Model file for the job. Use its own axes, mm. A direction names the side the tool comes from. Coordinates: 2 decimals unless noted, no trailing zeros. Order: outer loops, then holes, each group sorted by start corner. A loop starts at its lowest first (then second) coordinate and runs counter-clockwise, first axis right, second up. Notation, with made-up numbers: (59.5, 53) -> (66.5, 53) arc R25 ccw to (66.5, 71) -> close; hole circle Ø2 at (19, 50). An arc over 180 degrees is marked (long way). Use CSV: the item, a comma, the result in double quotes. Start each with the question number.
(1) Tool access for faces 1 (the cylindrical face through (-264, -40, 9)), 2 (the cylindrical face through (363.235, 38.668, 5.077)), 3 (the cylindrical face through (3.08, 2.64, 59.94)): list every direction of +Z, -Z, +X, -X, +Y, -Y with a clear straight run to the whole face (end or side of a thin tool).
(2) Probe L1, parallel to Y at x = 415, z = 0; L2, parallel to X at y = 4, z = -41; L3, parallel to Y at x = 417.25, z = 0. List the from-to ranges inside material, lowest first.
(3) Cut at B-B on x = 81.5. Write the cut outline in (y, z).
(4) Pin check, flat tips, straight feed: pin 1 Ø8 at (x, y) = (3, 16) entering from -Z; pin 2 Ø3 at (x, y) = (-96.5, -11.5) entering from -Z; pin 3 Ø5 at (x, z) = (-42, 21.5) entering from +Y. Stop position of each tip, or through.
(5) Cut at A-A on x = 280. Write the cut outline in (y, z).
```python
from build123d import *

# Parameters (mm, degrees)
SKETCH1_R           = 60
BOSS_EXTRUDE1_DEPTH = 220
SKETCH2_R           = 41
BOSS_EXTRUDE2_DEPTH = 310
SKETCH3_R           = 39
BOSS_EXTRUDE3_DEPTH = 420
SKETCH4_R           = 3.75
CUT_EXTRUDE1_DEPTH  = 6.25
SKETCH5_R           = 3.6
CUT_EXTRUDE2_DEPTH  = 6.25
CHAMFER1_SIZE       = 5


with BuildPart() as part:
    # Sketch1 → Boss-Extrude1 (new body, symmetric)
    with BuildSketch(Plane(origin=(0, 0, 0), x_dir=(0, 0, -1), z_dir=(1, 0, 0))):
        Circle(SKETCH1_R)
    extrude(amount=BOSS_EXTRUDE1_DEPTH, both=True)

    # Sketch2 → Boss-Extrude2 (add, symmetric)
    with BuildSketch(Plane(origin=(0, 0, 0), x_dir=(0, 0, -1), z_dir=(1, 0, 0))):
        Circle(SKETCH2_R)
    extrude(amount=BOSS_EXTRUDE2_DEPTH, both=True)

    # Sketch3 → Boss-Extrude3 (add, symmetric)
    with BuildSketch(Plane(origin=(0, 0, 0), x_dir=(0, 0, -1), z_dir=(1, 0, 0))):
        Circle(SKETCH3_R)
    extrude(amount=BOSS_EXTRUDE3_DEPTH, both=True)

    # Sketch4 → Cut-Extrude1 (cut)
    with BuildSketch(Plane(origin=(420, 0, 0), x_dir=(0, 0, -1), z_dir=(1, 0, 0))):
        Circle(SKETCH4_R)
    extrude(amount=-CUT_EXTRUDE1_DEPTH, mode=Mode.SUBTRACT)

    # Sketch5 → Cut-Extrude2 (cut)
    with BuildSketch(Plane.ZY.offset(420)):
        Circle(SKETCH5_R)
    extrude(amount=-CUT_EXTRUDE2_DEPTH, mode=Mode.SUBTRACT)

    # Chamfer1
    chamfer1_edges = [part.edges().sort_by_distance(p)[0] for p in [
        (-420, 0, 39),
        (420, 0, 39),
    ]]
    chamfer(chamfer1_edges, length=CHAMFER1_SIZE)


solid = part.part
```
Outcome:
1,face 1,"-X"
1,face 2,"+X"
1,face 3,"+X, -X"
2,L1,"-39 to -3.75, 3.75 to 39"
2,L2,"-220 to 220"
2,L3,"-36.75 to -3.75, 3.75 to 36.75"
3,outline,"circle Ø120 at (0, 0)"
4,pin 1,"z = -58.79"
4,pin 2,"z = -59.16"
4,pin 3,"y = 56.91"
5,outline,"circle Ø82 at (0, 0)"
